```python
from build123d import *

# Parameters (mm, degrees)
SKETCH1_W                                            = 56
SKETCH1_H                                            = 56
SKETCH1_W_2                                          = 27
SKETCH1_H_2                                          = 27
BOSS_EXTRUDE1_DEPTH                                  = 2
CHAMFER1_SIZE                                        = 1
CBORE_FOR_M3_CROSS_RECESS_PAN_HEAD_SCREW_D           = 3.4
CBORE_FOR_M3_CROSS_RECESS_PAN_HEAD_SCREW_DEPTH       = 5
CBORE_FOR_M3_CROSS_RECESS_PAN_HEAD_SCREW_CBORE_D     = 4.4
CBORE_FOR_M3_CROSS_RECESS_PAN_HEAD_SCREW_CBORE_DEPTH = 1
CBORE_FOR_M3_CROSS_RECESS_PAN_HEAD_SCREW_TIP         = 1.021463052
FILLET1_R                                            = 2


with BuildPart() as part:
    # Sketch1 → Boss-Extrude1 (new body)
    with BuildSketch(Plane(origin=(0, 0, 0), x_dir=(1, 0, 0), z_dir=(0, 1, 0))):
        with Locations((28, 28)):
            Rectangle(SKETCH1_W, SKETCH1_H)
        with Locations((28, 28)):
            Rectangle(SKETCH1_W_2, SKETCH1_H_2, mode=Mode.SUBTRACT)
    extrude(amount=BOSS_EXTRUDE1_DEPTH)

    # Chamfer1
    chamfer1_edges = [part.edges().sort_by_distance(p)[0] for p in [
        (14.5, 2, -28),
        (28, 2, -14.5),
        (41.5, 2, -28),
        (28, 2, -41.5),
    ]]
    chamfer(chamfer1_edges, length=CHAMFER1_SIZE)

    # CBORE for M3 Cross Recess Pan Head Screw1
    with Locations(Plane(origin=(0, 2, 0), x_dir=(1, 0, 0), z_dir=(0, 1, 0))):
        with Locations((9.461899873, 46.384256973), (46.794505385, 46.384256973), (46.794505385, 11.05161247), (9.820867233, 11.05161247)):
            CounterBoreHole(CBORE_FOR_M3_CROSS_RECESS_PAN_HEAD_SCREW_D / 2, CBORE_FOR_M3_CROSS_RECESS_PAN_HEAD_SCREW_CBORE_D / 2, CBORE_FOR_M3_CROSS_RECESS_PAN_HEAD_SCREW_CBORE_DEPTH, depth=CBORE_FOR_M3_CROSS_RECESS_PAN_HEAD_SCREW_DEPTH)
            with Locations((0, 0, -(CBORE_FOR_M3_CROSS_RECESS_PAN_HEAD_SCREW_DEPTH + CBORE_FOR_M3_CROSS_RECESS_PAN_HEAD_SCREW_TIP / 2))):  # 118° drill point
                Cone(0, CBORE_FOR_M3_CROSS_RECESS_PAN_HEAD_SCREW_D / 2, CBORE_FOR_M3_CROSS_RECESS_PAN_HEAD_SCREW_TIP, mode=Mode.SUBTRACT)

    # Fillet1
    fillet1_edges = [part.edges().sort_by_distance(p)[0] for p in [
        (0, 1, -56),
        (56, 1, -56),
        (56, 1, 0),
        (0, 1, 0),
    ]]
    fillet(fillet1_edges, radius=FILLET1_R)


solid = part.part
```
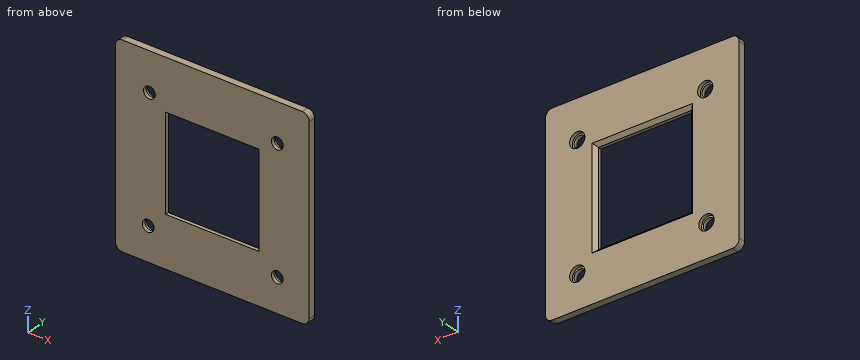
Check sheet for the modelled part. Datum: model origin and axes. Units: mm. Give positions to 0.01 mm unless a question says otherwise; leave off trailing zeros. Write each loop counter-clockwise with the first axis right and the second up, starting at its lowest first coordinate (ties: lowest second). Pieces come first, ordered by that corner, then holes. Notation, with made-up numbers: (-12, 9) - (47, 9) arc R7 cw to (47, 19) - close; hole circle Ø10 at (75.5, -17). An arc over 180 degrees is marked (long way). Answer as a JSON object with one key per item and string values. Group by question number.
1) Sectioned sample at C-C (y = 0.6). Record the cut outline in (x, z), then the cut area to 3 significant figures.
2) Depth check by flat-ended pin: P1, Ø2, axis at x = 9.5, z = -12, coming from the +Y side. Enter the tip coordinate at first touch or a pass-through.
3) Sectioned sample at B-B (x = 18). Record the cut outline in (y, z), then the cut area to 3 significant figures.
4) Sectioned sample at A-A (z = -27). Record the cut outline in (x, y), then the cut area to 3 significant figures.
5) Thickness scan on probe 1 along X at (y, z) = (1.6, -45); probe 2 along X at (y, z) = (0.3, -30.5); probe 3 along Z at (x, y) = (32, 0.7). Record the ranges inside material, lowest first. Write a range as from..to.
Geometry results:
{
 "1": {"outline": "(0, -54) arc R2 ccw to (2, -56) - (54, -56) arc R2 ccw to (56, -54) - (56, -2) arc R2 ccw to (54, 0) - (2, 0) arc R2 ccw to (0, -2) - close; hole circle Ø3.4 at (9.46, -46.38); hole circle Ø3.4 at (9.82, -11.05); hole (14.5, -41.5) - (41.5, -41.5) - (41.5, -14.5) - (14.5, -14.5) - close; hole circle Ø3.4 at (46.79, -46.38); hole circle Ø3.4 at (46.79, -11.05)", "area": "2,370 mm^2"},
 "2": {"P1": "stops at y = 1"},
 "3": {"outline": "(0, -56) - (2, -56) - (2, -42.5) - (1, -41.5) - (0, -41.5) - close; (0, -14.5) - (1, -14.5) - (2, -13.5) - (2, 0) - (0, 0) - close", "area": "57.0 mm^2"},
 "4": {"outline": "(0, 0) - (14.5, 0) - (14.5, 1) - (13.5, 2) - (0, 2) - close; (41.5, 0) - (56, 0) - (56, 2) - (42.5, 2) - (41.5, 1) - close", "area": "57.0 mm^2"},
 "5": {"probe 1": "x = 0..7.75, 11.17..45.08, 48.5..56", "probe 2": "x = 0..14.5, 41.5..56", "probe 3": "z = -56..-41.5, -14.5..0"}
}
